Could you check a few things on this drawing? It's one solid part, dimensions in mm from its lowest x, y, z. Give positions to 0.01 mm unless a question says otherwise; leave off trailing zeros. Loops run counter-clockwise (first coordinate to the right, second up) from the corner with the lowest first, then second, coordinate; pieces in that order, holes last. Notation, with made-up numbers: (85, 66.5) - (92, 66.5) arc R18 cw to (92, 96.5) - close; hole circle Ø8 at (82.25, -35.5). An arc over 180 degrees is marked (long way). Answer as a JSON object with one key per item and string values.
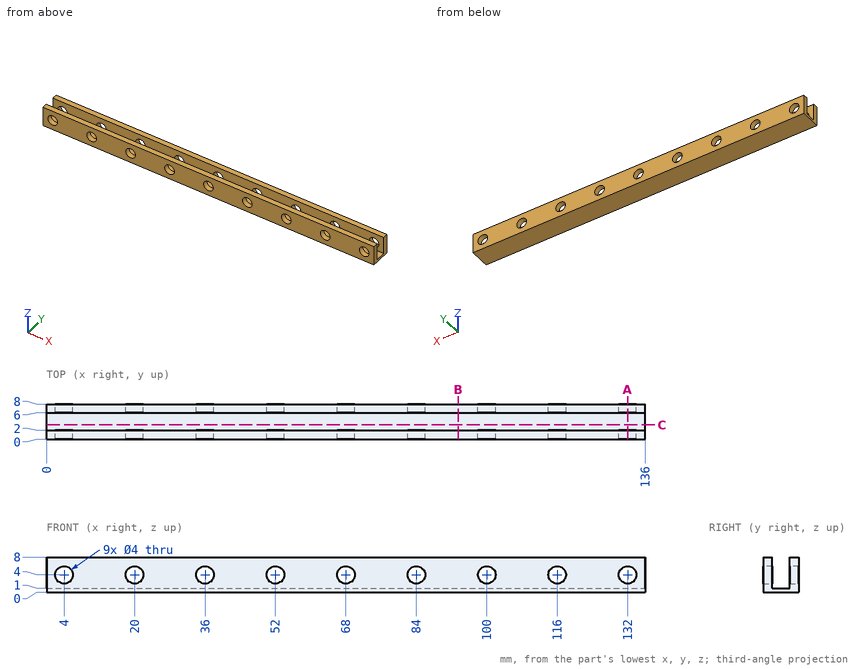
1) Imagine slicing it at B-B on x = 93.5. Write out the boundary of the cut face in (y, z), and give its area (3 significant figures).
Check sheet entries:
{"outline": "(0, 0) - (8, 0) - (8, 8) - (6, 8) - (6, 1) - (2, 1) - (2, 8) - (0, 8) - close", "area": "36.0 mm2"}
2) Imagine slicing it at C-C on y = 3.25. Write out the boundary of the cut face in (x, z).
Check sheet entries:
{"outline": "(0, 0) - (136, 0) - (136, 1) - (0, 1) - close"}
3) I need wall thicknesses on L1, parallel to Y at x = 110, z = 6.25; L2, parallel to Z at x = 25.5, y = 5. Which ranges of each line are inside material? Lowest first, please.
Check sheet entries:
{"L1": "0 to 2, 6 to 8", "L2": "0 to 1"}
4) Imagine slicing it at A-A on x = 132. Write out the boundary of the cut face in (y, z).
Check sheet entries:
{"outline": "(0, 0) - (8, 0) - (8, 2) - (6, 2) - (6, 1) - (2, 1) - (2, 2) - (0, 2) - close; (0, 6) - (2, 6) - (2, 8) - (0, 8) - close; (6, 6) - (8, 6) - (8, 8) - (6, 8) - close"}
5) I'm going to push flat-ended pins straight in: P1, Ø4.5, axis at x = 52, z = 4, coming from the +Y side; P2, Ø2.5, axis at x = 100, z = 4, coming from the -Y side. Where does each tip first touch, or does it pass through?
Check sheet entries:
{"P1": "y = 8", "P2": "through"}
